Input: part model. Units: mm. Frame: model coordinates. A direction names the side the tool comes from. Give positions to 0.01 mm unless a question says otherwise; leave off trailing zeros. Loops run counter-clockwise (first coordinate to the right, second up) from the corner with the lowest first, then second, coordinate; pieces in that order, holes last.
from build123d import *

# Parameters (mm, degrees)
CYLINDER017_R           = 1
CYLINDER017_DEPTH       = 10
CYLINDER017_ROLL_ANGLE  = 90
CYLINDER011_R           = 2
CYLINDER011_DEPTH       = 10
CYLINDER011_PITCH_ANGLE = 90
CYLINDER014_R           = 2
CYLINDER014_DEPTH       = 10
CYLINDER014_PITCH_ANGLE = 90
CYLINDER013_R           = 2
CYLINDER013_DEPTH       = 10
CYLINDER013_PITCH_ANGLE = 90
CYLINDER015_R           = 2
CYLINDER015_DEPTH       = 10
CYLINDER015_PITCH_ANGLE = 90
CYLINDER002_W           = 14
CYLINDER002_H           = 8
CYLINDER002_ANGLE       = 180
CYLINDER001_W           = 15
CYLINDER001_H           = 10
CYLINDER001_ANGLE       = 180
CYLINDER003_W           = 14
CYLINDER003_H           = 8
CYLINDER003_ANGLE       = 180
CYLINDER_W              = 15
CYLINDER_H              = 10
CYLINDER_ANGLE          = 180
BOX001_W                = 28
BOX001_H                = 21
BOX001_DEPTH            = 8
BOX_W                   = 30
BOX_H                   = 21
BOX_DEPTH               = 10
FUSION_PLACEMENT_ANGLE  = 180


with BuildPart() as cilindro017:
    # Cylinder017 → Cylinder017 (new body)
    with BuildSketch(Plane.XY):
        Circle(CYLINDER017_R)
    extrude(amount=CYLINDER017_DEPTH)


with BuildPart() as cilindro017_1:
    # Cylinder017 roll: moved
    add(cilindro017.part.rotate(Axis((0, 0, 0), (1, 0, 0)), CYLINDER017_ROLL_ANGLE))


with BuildPart() as cilindro017_2:
    # Cylinder017 placement: moved
    add(cilindro017_1.part.moved(Location((-14, 90, 38.5))))


with BuildPart() as cilindro011:
    # Cylinder011 → Cylinder011 (new body)
    with BuildSketch(Plane.XY):
        Circle(CYLINDER011_R)
    extrude(amount=CYLINDER011_DEPTH)


with BuildPart() as cilindro011_1:
    # Cylinder011 pitch: moved
    add(cilindro011.part.rotate(Axis((0, 0, 0), (0, 1, 0)), CYLINDER011_PITCH_ANGLE))


with BuildPart() as cilindro011_2:
    # Cylinder011 placement: moved
    add(cilindro011_1.part.moved(Location((-32, 72.5, 39.5))))


with BuildPart() as cilindro014:
    # Cylinder014 → Cylinder014 (new body)
    with BuildSketch(Plane.XY):
        Circle(CYLINDER014_R)
    extrude(amount=CYLINDER014_DEPTH)


with BuildPart() as cilindro014_1:
    # Cylinder014 pitch: moved
    add(cilindro014.part.rotate(Axis((0, 0, 0), (0, 1, 0)), CYLINDER014_PITCH_ANGLE))


with BuildPart() as cilindro014_2:
    # Cylinder014 placement: moved
    add(cilindro014_1.part.moved(Location((-6, 46.5, 39.5))))


with BuildPart() as cilindro013:
    # Cylinder013 → Cylinder013 (new body)
    with BuildSketch(Plane.XY):
        Circle(CYLINDER013_R)
    extrude(amount=CYLINDER013_DEPTH)


with BuildPart() as cilindro013_1:
    # Cylinder013 pitch: moved
    add(cilindro013.part.rotate(Axis((0, 0, 0), (0, 1, 0)), CYLINDER013_PITCH_ANGLE))


with BuildPart() as cilindro013_2:
    # Cylinder013 placement: moved
    add(cilindro013_1.part.moved(Location((-32, 46.5, 39.5))))


with BuildPart() as cilindro015:
    # Cylinder015 → Cylinder015 (new body)
    with BuildSketch(Plane.XY):
        Circle(CYLINDER015_R)
    extrude(amount=CYLINDER015_DEPTH)


with BuildPart() as cilindro015_1:
    # Cylinder015 pitch: moved
    add(cilindro015.part.rotate(Axis((0, 0, 0), (0, 1, 0)), CYLINDER015_PITCH_ANGLE))


with BuildPart() as cilindro015_2:
    # Cylinder015 placement: moved
    add(cilindro015_1.part.moved(Location((-5, 72.5, 39.5))))


with BuildPart() as cilindro002:
    # Cylinder002 → Cylinder002 (revolve)
    with BuildSketch(Plane(origin=(16, 49, -36), x_dir=(1, 0, 0), z_dir=(0, 1, 0))):
        with Locations((7, 4)):
            Rectangle(CYLINDER002_W, CYLINDER002_H)
    revolve(axis=Axis((16, 49, -36), (0, 0, -1)), revolution_arc=CYLINDER002_ANGLE)


with BuildPart() as cut001:
    # Cylinder001 → Cylinder001 (revolve)
    with BuildSketch(Plane(origin=(16, 49, -34), x_dir=(1, 0, 0), z_dir=(0, 1, 0))):
        with Locations((7.5, 5)):
            Rectangle(CYLINDER001_W, CYLINDER001_H)
    revolve(axis=Axis((16, 49, -34), (0, 0, -1)), revolution_arc=CYLINDER001_ANGLE)

    # Cut001: cut Cilindro002
    add(cilindro002.part, mode=Mode.SUBTRACT)


with BuildPart() as cut001_1:
    # Cut001 placement: moved
    add(cut001.part.moved(Location((-3, 0, 0))))


with BuildPart() as cilindro003:
    # Cylinder003 → Cylinder003 (revolve)
    with BuildSketch(Plane(origin=(13, 70, -36), x_dir=(-1, 0, 0), z_dir=(0, -1, 0))):
        with Locations((7, 4)):
            Rectangle(CYLINDER003_W, CYLINDER003_H)
    revolve(axis=Axis((13, 70, -36), (0, 0, -1)), revolution_arc=CYLINDER003_ANGLE)


with BuildPart() as cut002:
    # Cylinder → Cylinder (revolve)
    with BuildSketch(Plane(origin=(13, 70, -34), x_dir=(-1, 0, 0), z_dir=(0, -1, 0))):
        with Locations((7.5, 5)):
            Rectangle(CYLINDER_W, CYLINDER_H)
    revolve(axis=Axis((13, 70, -34), (0, 0, -1)), revolution_arc=CYLINDER_ANGLE)

    # Cut002: cut Cilindro003
    add(cilindro003.part, mode=Mode.SUBTRACT)


with BuildPart() as cubo001:
    # Box001 → Box001 (new body)
    with BuildSketch(Plane(origin=(-1, 49, -44), x_dir=(1, 0, 0), z_dir=(0, 0, 1))):
        with Locations((14, 10.5)):
            Rectangle(BOX001_W, BOX001_H)
    extrude(amount=BOX001_DEPTH)


with BuildPart() as cut025:
    # Box → Box (new body)
    with BuildSketch(Plane(origin=(-2, 49, -44), x_dir=(1, 0, 0), z_dir=(0, 0, 1))):
        with Locations((15, 10.5)):
            Rectangle(BOX_W, BOX_H)
    extrude(amount=BOX_DEPTH)

    # Cut: cut Cubo001
    add(cubo001.part, mode=Mode.SUBTRACT)

    # Fusion: union Cut001, Cut002
    add(cut001_1.part)
    add(cut002.part)


with BuildPart() as cut025_1:
    # Fusion placement: moved
    add(cut025.part.rotate(Axis((0, 0, 0), (0, 1, 0)), FUSION_PLACEMENT_ANGLE))

    # Cut021: cut Cilindro015
    add(cilindro015_2.part, mode=Mode.SUBTRACT)

    # Cut022: cut Cilindro013
    add(cilindro013_2.part, mode=Mode.SUBTRACT)

    # Cut023: cut Cilindro014
    add(cilindro014_2.part, mode=Mode.SUBTRACT)

    # Cut024: cut Cilindro011
    add(cilindro011_2.part, mode=Mode.SUBTRACT)

    # Cut025: cut Cilindro017
    add(cilindro017_2.part, mode=Mode.SUBTRACT)


solid = cut025_1.part
(1) Mould query, pull axis X, two halves, no side actions, for faces 4 (the flat face through (1.5, 61.5, 44)), 5 (the cylindrical face through (-12.67, 84.996, 39.07)), 6 (the flat face through (-13, 60, 36)), 7 (the flat face through (-28, 59, 39)). Classes: +X half, -X half, draft (parallel to the pull), parting line (faces both ways), or undercut.
Values follow:
face 4: draft
face 5: parting line
face 6: undercut
face 7: -X half
(2) Ray query, probe 1 along Z at (x, y) = (-14, 84); probe 2 along Z at (x, y) = (-27, 72.5); probe 3 along X at (y, z) = (69.5, 38.25). Return the intervals inside material, ascending.
Values follow:
probe 1: z = 34 to 37.5, 39.5 to 44
probe 2: z = 34 to 37.5, 41.5 to 44
probe 3: x = -28 to -27, 1 to 2
(3) Cut plane C-C (z = 38.5). Return the cut outline in (x, y).
Values follow:
outline: (-28, 49) arc R15 ccw to (-27.98, 48.23) - (-26.98, 48.23) arc R14 cw to (-27, 49) - (-27, 70) arc R14 cw to (-26.98, 70.77) - (-27.98, 70.77) arc R15 ccw to (-28, 70) - close; (-27.39, 44.77) arc R15 ccw to (1.39, 44.77) - (0.35, 44.77) arc R14 cw to (-26.35, 44.77) - close; (-27.39, 74.23) - (-26.35, 74.23) arc R14 cw to (-15, 83.86) - (-15, 84.87) arc R15 ccw to start; (-13, 84) arc R14 cw to (0.35, 74.23) - (1.39, 74.23) arc R15 ccw to (-13, 85) - close; (0.98, 48.23) - (1.98, 48.23) arc R15 ccw to (2, 49) - (2, 70) arc R15 ccw to (1.98, 70.77) - (0.98, 70.77) arc R14 cw to (1, 70) - (1, 49) arc R14 cw to start
(4) Cut plane B-B (x = -13.5). Return the cut outline in (y, z), and give its area (3 significant figures).
Values follow:
outline: (34.01, 34) - (84.99, 34) - (84.99, 37.63) - (83.99, 37.63) - (83.99, 36) - (35.01, 36) - (35.01, 44) - (34.01, 44) - close; (83.99, 39.37) - (84.99, 39.37) - (84.99, 44) - (83.99, 44) - close
area: 116 mm2
(5) Pin query (flat end, axial travel): pin 1 Ø3 at (x, z) = (-9.5, 41.5) entering from +Y; pin 2 Ø1.6 at (x, z) = (-14, 38.5) entering from +Y; pin 3 Ø5 at (x, z) = (-5.5, 36) entering from +Y; pin 4 Ø2.5 at (y, z) = (46.5, 39.5) entering from +X. Return the tip coordinate at first contact, or that it passes through.
Values follow:
pin 1: stops at y = 84.87
pin 2: stops at y = 35.12
pin 3: stops at y = 84.14
pin 4: passes through
(6) Cut plane A-A (y = 72.5). Return the cut outline in (x, z).
Values follow:
outline: (-27.79, 34) - (1.79, 34) - (1.79, 37.5) - (0.77, 37.5) - (0.77, 36) - (-26.77, 36) - (-26.77, 37.5) - (-27.79, 37.5) - close; (-27.79, 41.5) - (-26.77, 41.5) - (-26.77, 44) - (-27.79, 44) - close; (0.77, 41.5) - (1.79, 41.5) - (1.79, 44) - (0.77, 44) - close
(7) Reachability of faces 1 (the cylindrical face through (-27.137, 44.548, 39.934)), 2 (the cylindrical face through (-14.13, 84.44, 39.49)), 3 (the cylindrical face through (-13, 84, 40)) from +Z, -Z, +X, -X, +Y, -Y: full face, straight path, thin tool, end or side. Return the list, or none.
Values follow:
face 1: +X, -X
face 2: +Y
face 3: +Z
(8) Cut plane D-D (x = -25). Return the cut outline in (y, z).
Values follow:
outline: (40, 34) - (79, 34) - (79, 44) - (77.21, 44) - (77.21, 36) - (41.79, 36) - (41.79, 44) - (40, 44) - close
